```python
from build123d import *

# Parameters (mm, degrees)
BOSS_EXTRUDE1_DEPTH      = 1.5
BOSS_EXTRUDE1_DEPTH_BACK = 1.5
SKETCH3_W                = 10
SKETCH3_H                = 10.5
BOSS_EXTRUDE2_DEPTH      = 2


with BuildPart() as part:
    # Sketch1 → Boss-Extrude1 (new, two sides: drawn at the far end of the back side and taken through both)
    with BuildSketch(Plane(origin=(0, 0, 0), x_dir=(0, 0, -1), z_dir=(1, 0, 0)).offset(-BOSS_EXTRUDE1_DEPTH_BACK)):
        with BuildLine():
            Line((-5.460998077, 14.8), (-3.85, 14.8))
            ThreePointArc((-3.85, 14.8), (0, 8.75), (3.85, 14.8))
            Line((3.85, 14.8), (5.460998077, 14.8))
            ThreePointArc((5.460998077, 14.8), (5.747028676, 12.815171978), (5.334054451, 10.852824386))
            ThreePointArc((5.334054451, 10.852824386), (4.262621587, 5.434384876), (5.25, 0))
            Line((5.25, 0), (-5.25, 0))
            ThreePointArc((-5.25, 0), (-4.262621587, 5.434384876), (-5.334054451, 10.852824386))
            ThreePointArc((-5.334054451, 10.852824386), (-5.747028676, 12.815171978), (-5.460998077, 14.8))
        make_face()
    extrude(amount=BOSS_EXTRUDE1_DEPTH + BOSS_EXTRUDE1_DEPTH_BACK)

    # Sketch3 → Boss-Extrude2 (add)
    with BuildSketch(Plane.XZ):
        Rectangle(SKETCH3_W, SKETCH3_H)
    extrude(amount=-BOSS_EXTRUDE2_DEPTH)

    # Mirror1: part across plane


with BuildPart() as part_1:
    add(part.part)
    add(part.part.mirror(Plane(origin=(5, 2, -5.25), x_dir=(0, 0, 1), z_dir=(1, 0, 0))))


solid = part_1.part
```
Geometry check sheet. Reference: the model listing, model coordinates, mm. A direction names the side the tool comes from. Round coordinates to 2 decimals unless told otherwise and drop trailing zeros. Order: outer loops, then holes, each group sorted by start corner. A loop starts at its lowest first (then second) coordinate and runs counter-clockwise, first axis right, second up. Notation, with made-up numbers: (8, -13.5) - (59, -13.5) arc R19 ccw to (59, 3.5) - close; hole circle Ø11 at (-20.5, 37). An arc over 180 degrees is marked (long way). Use a Markdown table: item, result. Add a question column.
(1) Sectioned sample at C-C, the plane z = 0. Enter the section's corners in (x, y).
(2) Tool access check on faces 1 (the flat face through (11.5, 7, 0)), 2 (the flat face through (5, 1, 5.25)), 3 (the flat face through (5, 1, -5.25)). Record the directions out of +Z, -Z, +X, -X, +Y, -Y that give a thin tool (end or side, any length) a straight path to the whole face; none if there is none.
(3) Release check for a two-part mould opening along X. For faces 4 (the flat face through (5, 2, 0)), 5 (the cylindrical face through (10.021, 12.787, 5.746)), 6 (the flat face through (-1.5, 7, 0)) record: pulls with the +X half, pulls with the -X half, needs draft (parallel to the pull), parting line crosses it, or undercut.
(4) Sectioned sample at A-A, the plane y = 13. Enter the section's corners in (x, z).
(5) Sectioned sample at D-D, the plane x = -1. Enter the section's corners in (y, z).
(6) Sectioned sample at B-B, the plane y = 3.75. Enter the section's corners in (x, z), and give its area (3 significant figures).
(7) Depth check by flat-ended pin: pin 1 (5 mm diameter, centred on x = 0, z = 0, fed in from -Y); pin 2 (4 mm diameter, centred on x = 7.5, y = 8.5, fed in from +Z); pin 3 (3.5 mm diameter, centred on y = 10.5, z = -0.5, fed in from -X); pin 4 (0.6 mm diameter, centred on x = 8, y = 1, fed in from -Z). Enter the tip coordinate at first touch or a pass-through.
(8) Material ranges on line 1 along Z through (x, y) = (0.4, 13); line 2 along X through (y, z) = (12, 4.5); line 3 along Y through (x, z) = (1.75, -1), recorded low to high. Write a range as [from, to].
Answers below:
| question | item | result |
|---|---|---|
| 1 | outline | (-5, 0) - (15, 0) - (15, 2) - (11.5, 2) - (11.5, 8.75) - (8.5, 8.75) - (8.5, 2) - (1.5, 2) - (1.5, 8.75) - (-1.5, 8.75) - (-1.5, 2) - (-5, 2) - close |
| 2 | face 1 | +Z, -Z, +X, +Y |
| 2 | face 2 | +Z, +X, -X, -Y |
| 2 | face 3 | -Z, +X, -X, -Y |
| 3 | face 4 | undercut |
| 3 | face 5 | needs draft |
| 3 | face 6 | pulls with the -X half |
| 4 | outline | (-1.5, -5.75) - (1.5, -5.75) - (1.5, -4.25) - (-1.5, -4.25) - close; (-1.5, 4.25) - (1.5, 4.25) - (1.5, 5.75) - (-1.5, 5.75) - close; (8.5, -5.75) - (11.5, -5.75) - (11.5, -4.25) - (8.5, -4.25) - close; (8.5, 4.25) - (11.5, 4.25) - (11.5, 5.75) - (8.5, 5.75) - close |
| 5 | outline | (0, -5.25) - (2, -5.25) - (2, -4.64) arc R14.82 cw to (10.85, -5.33) arc R5.75 ccw to (14.8, -5.46) - (14.8, -3.85) arc R4.25 cw (long way) to (14.8, 3.85) - (14.8, 5.46) arc R5.75 ccw to (10.85, 5.33) arc R14.82 cw to (2, 4.64) - (2, 5.25) - (0, 5.25) - close |
| 6 | outline | (-1.5, -4.35) - (1.5, -4.35) - (1.5, 4.35) - (-1.5, 4.35) - close; (8.5, -4.35) - (11.5, -4.35) - (11.5, 4.35) - (8.5, 4.35) - close |
| 6 | area | 52.1 mm² |
| 7 | pin 1 | y = 0 |
| 7 | pin 2 | z = 5.1 |
| 7 | pin 3 | x = -1.5 |
| 7 | pin 4 | z = -5.25 |
| 8 | line 1 | [-5.75, -4.25], [4.25, 5.75] |
| 8 | line 2 | [-1.5, 1.5], [8.5, 11.5] |
| 8 | line 3 | [0, 2] |
